Read the model definition and answer for the solid it produces. Units are mm, in the model's axes. A direction names the side the tool comes from. Coordinates: 2 decimals unless noted, no trailing zeros. Order: outer loops, then holes, each group sorted by start corner. A loop starts at its lowest first (then second) coordinate and runs counter-clockwise, first axis right, second up. Notation, with made-up numbers: (34, 36) - (50, 36) arc R17 cw to (50, 54) - close; hole circle Ø10 at (50.5, 70.5). An arc over 180 degrees is marked (long way). Answer as a JSON object with one key per item and string values. Group by question number.
from build123d import *

# Parameters (mm, degrees)
F0_R     = 26.5
F0_R_2   = 1.2
F0_W     = 13
F0_H     = 8.5
F1_DEPTH = 2
F3_DEPTH = 6
F5_DEPTH = 1
F6_R     = 1.2
F7_DEPTH = 4


with BuildPart() as f1:
    # F0 (on Top) → F1 (new body)
    with BuildSketch(Plane.XY):
        Circle(F0_R)
        with Locations((-16.65, -16.65)):
            Circle(F0_R_2, mode=Mode.SUBTRACT)
        with Locations((16.65, -16.65)):
            Circle(F0_R_2, mode=Mode.SUBTRACT)
        with Locations((-15, 0)):
            Rectangle(F0_W, F0_H, mode=Mode.SUBTRACT)
        with Locations((-16.65, 16.65)):
            Circle(F0_R_2, mode=Mode.SUBTRACT)
        with Locations((16.65, 16.65)):
            Circle(F0_R_2, mode=Mode.SUBTRACT)
    extrude(amount=-F1_DEPTH)

    # F2 (on face) → F3 (join)
    with BuildSketch(Plane.XY):
        Polygon((23.5, 5.5), (-8.5, 5.5), (-8.5, 3.5), (21.5, 3.5), (21.5, -3.5), (-8.5, -3.5), (-8.5, -7.5), (23.5, -7.5), align=None)
    extrude(amount=F3_DEPTH)

    # F4 (on Right) → F5 (join, symmetric)
    with BuildSketch(Plane.YZ):
        Polygon((-26, 0), (-7.5, 0), (-7.5, 4), align=None)
        Polygon((5.5, 4), (5.5, 0), (26, 0), align=None)
    extrude(amount=F5_DEPTH, both=True)

    # F6 (on face) → F7 (cut, through all)
    with BuildSketch(Plane.XZ.offset(7.5)):
        with Locations((-4.5, 3)):
            Circle(F6_R)
        with Locations((17.5, 3)):
            Circle(F6_R)
    extrude(amount=-F7_DEPTH, mode=Mode.SUBTRACT)


solid = f1.part
1. Straight lines are drawn through the part: L1, parallel to Y at x = -16.65, z = -0.9; L2, parallel to Y at x = 11.5, z = 3; L3, parallel to Z at x = 6.5, y = 14. For each, find the intervals that lie inside material, in ascending order.
2. Given pin 1 (1 mm diameter, centred on x = 11, z = 4, fed in from +Y); pin 2 (1 mm diameter, centred on x = -7, y = 9, fed in from +Z); pin 3 (1.8 mm diameter, centred on x = 6.5, z = 3.5, fed in from -Y), each flat-ended and moving along its own axis, determine where each tip first touches the part or whether it passes through.
3. A cutting plane is placed at A-A on y = 0. Write down the section's boundary in (x, z).
4. For a pull along X with two mould halves and no side action, classify faces 4 (the flat face through (1, 11, 1)), 5 (the flat face through (21.5, 0, 3)), 6 (the cylindrical face through (16.3, -5.53, 3.05)), 7 (the flat face through (0, 0, -2)) as pulls with the +X half, pulls with the -X half, needs draft (parallel to the pull), parting line crosses it, or undercut.
5. A cutting plane is placed at C-C on z = -1. Write down the section's boundary in (x, y).
6. A cutting plane is placed at B-B on x = -12. Write down the section's boundary in (y, z), and give its area (3 significant figures).
7. A cutting plane is placed at D-D on x = 0. Write down the section's boundary in (y, z).
8. For faces 1 (the cylindrical face through (-5.7, -5.53, 3.05)), 2 (the flat face through (1, -13, 1)), 3 (the flat face through (-15, 4.25, -1)), determine the directions among +Z, -Z, +X, -X, +Y, -Y from which every point of the face is accessible in a straight line to the end or side of a thin tool.
Derived:
{
 "1": {"L1": "y = -20.62 to -17.85, -15.45 to -4.25, 4.25 to 15.45, 17.85 to 20.62", "L2": "y = -7.5 to -3.5, 3.5 to 5.5", "L3": "z = -2 to 0"},
 "2": {"pin 1": "stops at y = 5.5", "pin 2": "stops at z = 0", "pin 3": "stops at y = -7.5"},
 "3": {"outline": "(-26.5, -2) - (-21.5, -2) - (-21.5, 0) - (-26.5, 0) - close; (-8.5, -2) - (26.5, -2) - (26.5, 0) - (23.5, 0) - (23.5, 6) - (21.5, 6) - (21.5, 0) - (-8.5, 0) - close"},
 "4": {"face 4": "pulls with the +X half", "face 5": "pulls with the -X half", "face 6": "undercut", "face 7": "needs draft"},
 "5": {"outline": "circle Ø53 at (0, 0); hole (-21.5, -4.25) - (-8.5, -4.25) - (-8.5, 4.25) - (-21.5, 4.25) - close; hole circle Ø2.4 at (-16.65, -16.65); hole circle Ø2.4 at (-16.65, 16.65); hole circle Ø2.4 at (16.65, -16.65); hole circle Ø2.4 at (16.65, 16.65)"},
 "6": {"outline": "(-23.63, -2) - (-4.25, -2) - (-4.25, 0) - (-23.63, 0) - close; (4.25, -2) - (23.63, -2) - (23.63, 0) - (4.25, 0) - close", "area": "77.5 mm2"},
 "7": {"outline": "(-26.5, -2) - (26.5, -2) - (26.5, 0) - (26, 0) - (5.5, 4) - (5.5, 6) - (3.5, 6) - (3.5, 0) - (-3.5, 0) - (-3.5, 6) - (-7.5, 6) - (-7.5, 4) - (-26, 0) - (-26.5, 0) - close"},
 "8": {"face 1": "-Y", "face 2": "+Z, +X, -Y", "face 3": "+Z, -Z"}
}
